Part model, mm, in its own coordinate system. Face numbers are marked on the shaded views. A direction names the side the tool comes from. Give positions to 0.01 mm unless a question says otherwise; leave off trailing zeros. Write each loop counter-clockwise with the first axis right and the second up, starting at its lowest first coordinate (ties: lowest second). Pieces come first, ordered by that corner, then holes.
from build123d import *

# Parameters (mm, degrees)
BOSS_EXTRUDE1_DEPTH     = 9.75
SKETCH2_R               = 2.1
CUT_EXTRUDE1_DEPTH      = 27.914459404
CUT_EXTRUDE2_DEPTH      = 33.696722039
CUT_EXTRUDE2_DEPTH_BACK = 33.696722039


with BuildPart() as part:
    # Sketch1 → Boss-Extrude1 (new, symmetric)
    with BuildSketch(Plane(origin=(0, 0, 0), x_dir=(0, 0, -1), z_dir=(1, 0, 0))):
        with BuildLine():
            Line((-15.875, -16), (-15.875, 16))
            Line((-15.875, 16), (-7, 20.9))
            Line((-7, 20.9), (-2, 20.9))
            Line((-2, 20.9), (-2, 19.412087811))
            ThreePointArc((-2, 19.412087811), (-9.5, 10.125), (-2, 0.837912189))
            Line((-2, 0.837912189), (-2, -0.837912189))
            ThreePointArc((-2, -0.837912189), (-9.5, -10.125), (-2, -19.412087811))
            Line((-2, -19.412087811), (-2, -20.9))
            Line((-2, -20.9), (-7, -20.9))
            Line((-7, -20.9), (-15.875, -16))
        make_face()
    extrude(amount=BOSS_EXTRUDE1_DEPTH, both=True)

    # Sketch2 → Cut-Extrude1 (cut, through all)
    with BuildSketch(Plane.XY.offset(15.875)):
        with Locations((0, 10.125)):
            Circle(SKETCH2_R)
        with Locations((0, -10.125)):
            Circle(SKETCH2_R)
    extrude(amount=-CUT_EXTRUDE1_DEPTH, mode=Mode.SUBTRACT)

    # Sketch3 → Cut-Extrude2 (cut, two sides: drawn at the far end of the back side and taken through both)
    with BuildSketch(Plane.ZY.offset(9.75).offset(-CUT_EXTRUDE2_DEPTH_BACK)):
        with BuildLine():
            Line((15.875, 6), (12.375, 6))
            ThreePointArc((12.375, 6), (10.607233047, 5.267766953), (9.875, 3.5))
            Line((9.875, 3.5), (9.875, -3.5))
            ThreePointArc((9.875, -3.5), (10.607233047, -5.267766953), (12.375, -6))
            Line((12.375, -6), (15.875, -6))
            Line((15.875, -6), (15.875, 6))
        make_face()
    extrude(amount=CUT_EXTRUDE2_DEPTH + CUT_EXTRUDE2_DEPTH_BACK, mode=Mode.SUBTRACT)


solid = part.part
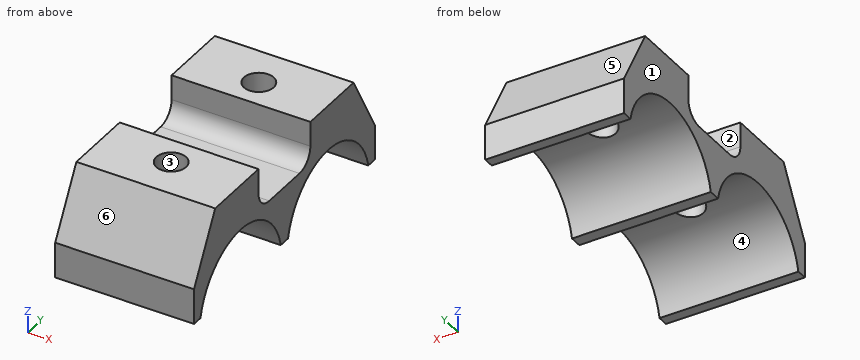
1) Saw through at A-A (x = 0). Write the cut outline in (y, z) (3 decimals).
Check result:
outline: (-20.9, 2) - (-19.412, 2) arc R9.5 cw to (-12.225, 9.265) - (-12.225, 15.875) - (-16, 15.875) - (-20.9, 7) - close; (-8.025, 9.265) arc R9.5 cw to (-0.838, 2) - (0.838, 2) arc R9.5 cw to (8.025, 9.265) - (8.025, 15.875) - (6, 15.875) - (6, 12.375) arc R2.5 cw to (3.5, 9.875) - (-3.5, 9.875) arc R2.5 cw to (-6, 12.375) - (-6, 15.875) - (-8.025, 15.875) - close; (12.225, 9.265) arc R9.5 cw to (19.412, 2) - (20.9, 2) - (20.9, 7) - (16, 15.875) - (12.225, 15.875) - close
2) Saw through at C-C (z = 13.75). Write the cut outline in (x, y) (3 decimals).
Check result:
outline: (-9.75, -17.173) - (9.75, -17.173) - (9.75, -6) - (-9.75, -6) - close; (-9.75, 6) - (9.75, 6) - (9.75, 17.173) - (-9.75, 17.173) - close; hole circle Ø4.2 at (0, -10.125); hole circle Ø4.2 at (0, 10.125)
3) Saw through at D-D (x = -6.25). Write the cut outline in (y, z) (3 decimals).
Check result:
outline: (-20.9, 2) - (-19.412, 2) arc R9.5 cw to (-0.838, 2) - (0.838, 2) arc R9.5 cw to (19.412, 2) - (20.9, 2) - (20.9, 7) - (16, 15.875) - (6, 15.875) - (6, 12.375) arc R2.5 cw to (3.5, 9.875) - (-3.5, 9.875) arc R2.5 cw to (-6, 12.375) - (-6, 15.875) - (-16, 15.875) - (-20.9, 7) - close
4) Mould opens along Y. For the marked faces 3, 4, 5 and 6 say: +Y half, -Y half, draft (parallel to the pull), parting line (faces both ways), or undercut.
Check result:
face 3: undercut
face 4: undercut
face 5: +Y half
face 6: -Y half
5) Flat gauge pins, fed straight in: P1, Ø7.5, axis at x = 2, y = -0.5, coming from the +Z side; P2, Ø4, axis at x = 2.5, z = 14.5, coming from the +Y side; P3, Ø5.5, axis at x = 0, y = 10.125, coming from the -Z side. Where does each tip first touch, or does it go through?
Check result:
P1: stops at z = 9.99
P2: stops at y = 17.86
P3: stops at z = 9.09
6) 3-axis set-ups, long thin cutter, end or side, ignore diameter. For the marked faces 1 and 2: which of +Z, -Z, +X, -X, +Y, -Y reach the whole face in a straight line?
Check result:
face 1: +Z, -Z, -X, +Y, -Y
face 2: +Z, +X, -X
7) Saw through at B-B (z = 3.5). Write the cut outline in (x, y), and give its area (3 significant figures).
Check result:
outline: (-9.75, -20.9) - (9.75, -20.9) - (9.75, -18.96) - (-9.75, -18.96) - close; (-9.75, -1.29) - (9.75, -1.29) - (9.75, 1.29) - (-9.75, 1.29) - close; (-9.75, 18.96) - (9.75, 18.96) - (9.75, 20.9) - (-9.75, 20.9) - close
area: 126 mm2
8) Drill centre lines: L1, parallel to Y at x = 0, z = 14 (3 decimals); L2, parallel to Y at x = 0, z = 12 (3 decimals); L3, parallel to Y at x = -1.25, z = 6.25. Where is each one in solid material? Low to high.
Check result:
L1: y = -17.035 to -12.225, -8.025 to -6, 6 to 8.025, 12.225 to 17.035
L2: y = -18.139 to -12.225, -8.025 to -5.972, 5.972 to 8.025, 12.225 to 18.139
L3: y = -20.9 to -17.28, -2.97 to 2.97, 17.28 to 20.9
